For this review, take the finished solid that the model builds, in its own axes (mm). A direction names the side the tool comes from. Round coordinates to 2 decimals unless told otherwise and drop trailing zeros. Order: outer loops, then holes, each group sorted by start corner. A loop starts at its lowest first (then second) coordinate and runs counter-clockwise, first axis right, second up. Notation, with made-up numbers: (32.5, 81) - (71.5, 81) arc R31 ccw to (71.5, 105) - close; hole circle Ø8 at (38, 51). An arc over 180 degrees is marked (long way). One line per item, written item: value.
```python
from build123d import *

# Parameters (mm, degrees)
SKETCH_1_R               = 70
SKETCH_1_R_2             = 35
EXTRUDE_1_DEPTH          = 10
SKETCH_1_3_R             = 35
SKETCH_1_3_R_2           = 25
EXTRUDE_2_DEPTH          = 50
RIB_13_REACH             = 112.905
SKETCH_2_WALL_W          = 273.614682576
SKETCH_2_WALL_H          = 10
PATTERN_CIRCULAR_1_COUNT = 3


with BuildPart() as part:
    # Sketch 1 → Extrude 1 (new body)
    with BuildSketch(Plane(origin=(0, 0, 0), x_dir=(1, 0, 0), z_dir=(0, 1, 0))):
        with Locations(Location((0, 0, 0), (0, 0, 270))):
            Circle(SKETCH_1_R)
        with Locations(Location((0, 0, 0), (0, 0, 270))):
            Circle(SKETCH_1_R_2, mode=Mode.SUBTRACT)
    extrude(amount=EXTRUDE_1_DEPTH)

    # Sketch 1_3 → Extrude 2 (add)
    with BuildSketch(Plane(origin=(0, 0, 0), x_dir=(1, 0, 0), z_dir=(0, 1, 0))):
        with Locations(Location((0, 0, 0), (0, 0, 270))):
            Circle(SKETCH_1_3_R)
        with Locations(Location((0, 0, 0), (0, 0, 270))):
            Circle(SKETCH_1_3_R_2, mode=Mode.SUBTRACT)
    extrude(amount=EXTRUDE_2_DEPTH)

    # Sketch 2 wall → Rib 13 (add, up to next)
    with BuildSketch(Plane(origin=(0, 28.909855829, 51.202647079), x_dir=(0, -0.7593716924, 0.650657077716), z_dir=(0, -0.650657077716, -0.7593716924)), mode=Mode.PRIVATE) as rib_13_sk1:
        Rectangle(SKETCH_2_WALL_W, SKETCH_2_WALL_H)
    rib_13_tool1 = extrude(rib_13_sk1.sketch, amount=RIB_13_REACH, mode=Mode.PRIVATE) - part.part
    rib_13 = rib_13_tool1.solids().sort_by_distance((0, 28.909855829, 51.202647079))[0]
    add(rib_13)

    # Pattern Circular 1: Rib 13 ×3 about axis
    pattern_circular_1_axis = Axis((0, 0, 0), (0, 1, 0))
    for i in range(1, PATTERN_CIRCULAR_1_COUNT):
        add(rib_13.rotate(pattern_circular_1_axis, i * 360 / PATTERN_CIRCULAR_1_COUNT))


solid = part.part
```
Item 1: Take a section at A-A (x = 21). Write out the cut boundary in (y, z), plus the area to 3 significant figures.
Returned:
outline: (0, -66.78) - (10, -66.78) - (10, -28) - (50, -28) - (50, -13.56) - (0, -13.56) - close; (0, 13.56) - (50, 13.56) - (50, 28) - (10, 28) - (10, 66.78) - (0, 66.78) - close
area: 2,220 mm^2
Item 2: Take a section at B-B (z = 0). Write out the cut boundary in (x, y), plus the area to 3 significant figures.
Returned:
outline: (-70, 0) - (-25, 0) - (-25, 50) - (-35, 50) - (-35, 10) - (-70, 10) - close; (25, 0) - (70, 0) - (70, 10) - (35, 10) - (35, 50) - (25, 50) - close
area: 1,700 mm^2
Item 3: Wall thickness on line 1 (X direction, y = 30, z = 0); line 2 (Y direction, x = 39.5, z = 16.5); line 3 (X direction, y = 39.5, z = -17.5): over which ranges is each line inside the solid? List them lowest first.
Returned:
line 1: -35 to -25, 25 to 35
line 2: 0 to 10
line 3: -38.54 to -17.85, 17.85 to 38.54
Item 4: Take a section at C-C (y = 44.5). Write out the cut boundary in (x, z), plus the area to 3 significant figures.
Returned:
outline: (-35.27, -14.59) - (-30.27, -23.25) - (-27.5, -21.65) arc R35 ccw to (27.5, -21.65) - (30.27, -23.25) - (35.27, -14.59) - (32.5, -12.99) arc R35 ccw to (5, 34.64) - (5, 37.84) - (-5, 37.84) - (-5, 34.64) arc R35 ccw to (-32.5, -12.99) - close; hole circle Ø50 at (0, 0)
area: 1,970 mm^2
Item 5: For P1, Ø1, axis at y = 45, z = 7.5, coming from the -X side; P2, Ø5, axis at x = -26, y = 27.5, coming from the +Z side; P3, Ø6, axis at x = 42, y = 21, coming from the -Z side; P4, Ø10, axis at x = 49, y = 42.5, coming from the +Z side, all flat-tipped, find the tip position at first contact; note any pin that passes through.
Returned:
P1: x = -34.29
P2: z = 25.94
P3: z = -31.75
P4: through
Item 6: Machinability: for faces 1 (the flat face through (5, 25, 46)), 2 (the flat face through (-42.06, 25, -18.51)), 3 (the flat face through (37.06, 25, -27.17)), which of the approach directions +Z, -Z, +X, -X, +Y, -Y give a long, thin tool a straight path to every point of the face, cutting with its end or side? Answer none if there is none.
Returned:
face 1: +Z, +X, +Y
face 2: -X, +Y
face 3: -Z, +Y
Item 7: Take a section at D-D (z = 49). Write out the cut boundary in (x, y).
Returned:
outline: (-49.99, 0) - (49.99, 0) - (49.99, 10) - (5, 10) - (5, 31.48) - (-5, 31.48) - (-5, 10) - (-49.99, 10) - close
Item 8: The part is to be moulded in two halves that separate along X. For faces 4 (the flat face through (-37.06, 25, -27.17)), 5 (the flat face through (8, 50, -24)), 6 (the cylindrical face through (-42.594, 4.93, -55.55)), say which applies: +X half, -X half, draft (parallel to the pull), parting line (faces both ways), or undercut.
Returned:
face 4: undercut
face 5: draft
face 6: parting line
